Source: CAD feature listing. Evaluate the final solid. Frame: model axes, mm. A direction names the side the tool comes from. Coordinates: 2 decimals unless noted, no trailing zeros. Order: outer loops, then holes, each group sorted by start corner. A loop starts at its lowest first (then second) coordinate and runs counter-clockwise, first axis right, second up. Notation, with made-up numbers: (-0.75, 8.5) - (10.25, 8.5) arc R28 cw to (10.25, 34.5) - close; hole circle Ø4 at (26.25, 6). An arc over 180 degrees is marked (long way). One line per question, with ' | ' between items. Start each with the question number.
(1) Contact query for flat-ended pins moving along their axis: P1, Ø1, axis at x = -1.5, y = -2.5, coming from the -Z side; P2, Ø5, axis at y = -4.5, z = 1, coming from the +X side; P3, Ø2, axis at y = -2, z = 4, coming from the -X side. Output: stop coordinate, or through.
(2) Line query: line 1 along Z through (x, y) = (-0.5, -2.5); line 2 along Z through (x, y) = (0, -7.5); line 3 along X through (y, z) = (-3, 4.75). Output: solid intervals per line, ascending.
(3) Section D-D (x = 2.25). Return the cut outline in (y, z).
(4) Section A-A (x = 0). Return the cut outline in (y, z).
(5) Section B-B (z = 0). Return the cut outline in (x, y), then the cut area to 3 significant figures.
(6) Draft query along X for faces 1 (the flat face through (2.585, -2.958, 5.109)), 2 (the flat face through (-1.506, -3.042, 5.624)), 3 (the cylindrical face through (-0.08, -2.96, -3.25)), 4 (the cylindrical face through (0, -3, 3.6)). Return one class per face: +X half, -X half, draft (parallel to the pull), parting line (faces both ways), or undercut.
(7) Section C-C (y = -4.75). Return the cut outline in (x, z), then the cut area to 3 significant figures.
(8) Access query for faces 5 (the cylindrical face through (1.813, -2.958, -1.059)), 6 (the flat face through (-2.567, -2.958, 5.242)). Directions: +Z, -Z, +X, -X, +Y, -Y. A direction counts if a zero-diameter tool reaches every point of the face in a straight line with its end or side. Return the directions, or none.
from build123d import *

# Parameters (mm, degrees)
F0_R     = 2.1
F0_R_2   = 1.05
F1_DEPTH = 6
F3_DEPTH = 25
F5_DEPTH = 25
F6_R     = 1.95
F6_R_2   = 1.05
F7_DEPTH = 4


with BuildPart() as f1:
    # F0 (on Front) → F1 (new body)
    with BuildSketch(Plane.XZ):
        with BuildLine():
            Line((-1.9322245482, 9.9126943005), (-3.2203742469, 0.4378238342))
            ThreePointArc((-3.2203742469, 0.4378238342), (0, -3.25), (3.2203742469, 0.4378238342))
            Line((3.2203742469, 0.4378238342), (1.9322245482, 9.9126943005))
            ThreePointArc((1.9322245482, 9.9126943005), (0, 11.6), (-1.9322245482, 9.9126943005))
        make_face()
        Circle(F0_R, mode=Mode.SUBTRACT)
        with Locations((0, 9.65)):
            Circle(F0_R_2, mode=Mode.SUBTRACT)
    extrude(amount=F1_DEPTH)

    # F2 (on face) → F3 (cut)
    with BuildSketch(Plane.XZ.offset(6)):
        with BuildLine():
            ThreePointArc((1.170751587, 8.0905639733), (0, 7.7), (-1.170751587, 8.0905639733))
            Line((-1.170751587, 8.0905639733), (-1.850907083, 3.087740755))
            ThreePointArc((-1.850907083, 3.087740755), (0, 3.6), (1.850907083, 3.087740755))
            Line((1.850907083, 3.087740755), (1.170751587, 8.0905639733))
        make_face()
    extrude(amount=-F3_DEPTH, mode=Mode.SUBTRACT)

    # F4 (on face) → F5 (cut)
    with BuildSketch(Plane.XZ.offset(6)):
        with BuildLine():
            Line((-0.75, 1.9615045246), (-0.75, 2.3848480035))
            ThreePointArc((-0.75, 2.3848480035), (-2.1650635095, 1.25), (-2.4403389552, -0.5429049489))
            Line((-2.4403389552, -0.5429049489), (-2.0737127479, -0.3312332095))
            ThreePointArc((-2.0737127479, -0.3312332095), (-1.8186533479, 1.05), (-0.75, 1.9615045246))
        make_face()
        with BuildLine():
            ThreePointArc((1.3237127479, -1.6302713151), (0, -2.1), (-1.3237127479, -1.6302713151))
            Line((-1.3237127479, -1.6302713151), (-1.6903389552, -1.8419430546))
            ThreePointArc((-1.6903389552, -1.8419430546), (0, -2.5), (1.6903389552, -1.8419430546))
            Line((1.6903389552, -1.8419430546), (1.3237127479, -1.6302713151))
        make_face()
        with BuildLine():
            ThreePointArc((0.75, 1.9615045246), (1.8186533479, 1.05), (2.0737127479, -0.3312332095))
            Line((2.0737127479, -0.3312332095), (2.4403389552, -0.5429049489))
            ThreePointArc((2.4403389552, -0.5429049489), (2.1650635095, 1.25), (0.75, 2.3848480035))
            Line((0.75, 2.3848480035), (0.75, 1.9615045246))
        make_face()
    extrude(amount=-F5_DEPTH, mode=Mode.SUBTRACT)

    # F6 (on face) → F7 (join)
    with BuildSketch(Plane.XZ.offset(6)):
        with Locations((0, 9.65)):
            Circle(F6_R)
        with Locations((0, 9.65)):
            Circle(F6_R_2, mode=Mode.SUBTRACT)
    extrude(amount=F7_DEPTH)


solid = f1.part
Response values:
1) P1: stops at z = -3.09 | P2: stops at x = 3.25 | P3: stops at x = -2.87
2) line 1: z = -3.21 to -2.45, 2.04 to 3.57, 7.77 to 8.73, 10.57 to 11.53 | line 2: z = 7.7 to 8.6, 10.7 to 11.6 | line 3: x = -2.63 to -1.62, 1.62 to 2.63
3) outline: (-6, -2.35) - (0, -2.35) - (0, -0.43) - (-6, -0.43) - close; (-6, 1.09) - (0, 1.09) - (0, 7.58) - (-6, 7.58) - close
4) outline: (-10, 7.7) - (0, 7.7) - (0, 8.6) - (-10, 8.6) - close; (-10, 10.7) - (0, 10.7) - (0, 11.6) - (-10, 11.6) - close; (-6, -3.25) - (0, -3.25) - (0, -2.5) - (-6, -2.5) - close; (-6, 2.1) - (0, 2.1) - (0, 3.6) - (-6, 3.6) - close
5) outline: (-3.25, -6) - (-2.5, -6) - (-2.5, 0) - (-3.25, 0) - close; (2.5, -6) - (3.25, -6) - (3.25, 0) - (2.5, 0) - close | area: 9.00 mm²
6) face 1: +X half | face 2: undercut | face 3: parting line | face 4: undercut
7) outline: (-3.22, 0.44) arc R3.25 ccw (long way) to (3.22, 0.44) - (1.93, 9.91) arc R1.95 ccw to (-1.93, 9.91) - close; hole (-2.44, -0.54) - (-2.07, -0.33) arc R2.1 ccw to (-1.32, -1.63) - (-1.69, -1.84) arc R2.5 ccw to (1.69, -1.84) - (1.32, -1.63) arc R2.1 ccw to (2.07, -0.33) - (2.44, -0.54) arc R2.5 ccw to (0.75, 2.38) - (0.75, 1.96) arc R2.1 ccw to (-0.75, 1.96) - (-0.75, 2.38) arc R2.5 ccw to start; hole (-1.85, 3.09) arc R3.6 cw to (1.85, 3.09) - (1.17, 8.09) arc R1.95 cw to (-1.17, 8.09) - close; hole circle Ø2.1 at (0, 9.65) | area: 38.7 mm²
8) face 5: +Y, -Y | face 6: +Z, -X, +Y, -Y
